Model file for the job. Use its own axes, mm. A direction names the side the tool comes from. Give positions to 0.01 mm unless a question says otherwise; leave off trailing zeros. Write each loop counter-clockwise with the first axis right and the second up, starting at its lowest first coordinate (ties: lowest second). Pieces come first, ordered by that corner, then holes. Notation, with made-up numbers: (-6.5, -26) - (38.5, -26) arc R13 ccw to (38.5, -11) - close; hole circle Ø5 at (55.5, 45.5). An arc over 180 degrees is marked (long way). Use CSV: the item, a comma, the result in double quotes.
from build123d import *

# Parameters (mm, degrees)
F0_W     = 190.5
F0_H     = 12.7
F1_DEPTH = 38.1
F2_W     = 165.1
F2_H     = 25.4
F3_DEPTH = 12.701
F4_R     = 6.34999


# Not quite as in the source:
# - a fillet or chamfer is up to 0.001 mm smaller than in the source, because OpenCascade refuses the exact size


with BuildPart() as f1:
    # F0 (on Front) → F1 (new body)
    with BuildSketch(Plane.XZ):
        Rectangle(F0_W, F0_H)
    extrude(amount=F1_DEPTH)

    # F2 (on face) → F3 (cut, through all)
    with BuildSketch(Plane.XY.offset(6.35)):
        with Locations((0, -12.7)):
            Rectangle(F2_W, F2_H)
    extrude(amount=-F3_DEPTH, mode=Mode.SUBTRACT)

    # F4 (radius 6.35 in the source; OpenCascade refuses exactly that, so slightly less here)
    f4_edges = [f1.edges().sort_by_distance(p)[0] for p in [
        (-95.25, -38.1, 0),
        (-82.55, -25.4, 0),
        (95.25, -38.1, 0),
        (82.55, -25.4, 0),
        (0, -38.1, 6.35),
        (0, -25.4, 6.35),
        (0, -38.1, -6.35),
        (0, -25.4, -6.35),
        (-82.55, -12.7, -6.35),
        (-95.25, -19.05, -6.35),
        (82.55, -12.7, -6.35),
        (95.25, -19.05, -6.35),
        (95.25, -19.05, 6.35),
        (-82.55, -12.7, 6.35),
        (-95.25, -19.05, 6.35),
        (82.55, -12.7, 6.35),
    ]]
    fillet(f4_edges, radius=F4_R)


solid = f1.part
(1) Saw through at C-C, the plane z = -3.25. List the corners of the cut face in (x, y), then the cut area to 3 significant figures.
Checked values:
outline,"(-94.36, -31.75) arc R5.46 ccw to (-88.9, -37.21) - (88.9, -37.21) arc R5.46 ccw to (94.36, -31.75) - (94.36, 0) - (83.44, 0) - (83.44, -19.05) arc R7.24 cw to (76.2, -26.29) - (-76.2, -26.29) arc R7.24 cw to (-83.44, -19.05) - (-83.44, 0) - (-94.36, 0) - close"
area,"2,640 mm^2"
(2) Flat gauge pins, fed straight in: P1, Ø6, axis at y = -4, z = 3.5, coming from the -X side; P2, Ø6, axis at x = 29, y = -27.5, coming from the -Z side; P3, Ø3, axis at y = -7.5, z = -4, coming from the -X side; P4, Ø12, axis at x = -21, y = -19, coming from the +Z side. Where does each tip first touch, or does it go through?
Checked values:
P1,"stops at x = -95.23"
P2,"stops at z = -6.23"
P3,"stops at x = -94.74"
P4,"passes through"
(3) 3-axis set-ups, long thin cutter, end or side, ignore diameter. For faces 4 (the face through (1.07, -27.31, 4.54)), 5 (the face through (-84.46, -9.39, -4.54)), 6 (the face through (93.34, -16.1, 4.54)): which of +Z, -Z, +X, -X, +Y, -Y reach the whole face in a straight line?
Checked values:
face 4,"+Z, +Y"
face 5,"-Z, +Y"
face 6,"+Z, +X, +Y, -Y"
(4) Pull direction X, two halves, no side cores. Call faces 1 (the face through (-93.44, -16.1, 4.44)), 2 (the face through (84.46, -9.39, 4.54)), 3 (the face through (1.24, -36.19, -4.54)): released by +X, released by -X, zero draft, split by the parting line, or undercut.
Checked values:
face 1,"released by -X"
face 2,"undercut"
face 3,"zero draft"
(5) Wall check: probe 1 along X at (y, z) = (-32, 0); probe 2 along X at (y, z) = (-9, -0.5); probe 3 along Z at (x, y) = (-47, -32). Give the ranges that are in metal, low to high. Write a range as [from, to].
Checked values:
probe 1,"x = [-95.25, 95.25]"
probe 2,"x = [-95.23, -82.57], [82.57, 95.23]"
probe 3,"z = [-6.35, 6.35]"
